```python
from build123d import *

# Parameters (mm, degrees)
CROQUIS1_W                = 139.5
CROQUIS1_H                = 83
SALIENTE_EXTRUIR1_DEPTH   = 27.5
CORTAR_EXTRUIR1_START     = -66.254131909
CORTAR_EXTRUIR1_OUTLINE_W = 22
CORTAR_EXTRUIR1_OUTLINE_H = 80
CORTAR_EXTRUIR1_DEPTH     = 132.508263818
CORTAR_EXTRUIR2_DEPTH     = 40
CROQUIS6_W                = 30
CROQUIS6_H                = 13.5
CROQUIS6_W_2              = 16.5
CORTAR_EXTRUIR3_DEPTH     = 3.495868091
CROQUIS7_R                = 2.5
CROQUIS7_W                = 21
CROQUIS7_H                = 30
CORTAR_EXTRUIR4_DEPTH     = 85.85207717


# Read off the part's stored shape, not the designer's step: Cortar-Extruir1
with BuildPart() as part:
    # Croquis1 → Saliente-Extruir1 (new body)
    with BuildSketch(Plane(origin=(0, 0, 0), x_dir=(1, 0, 0), z_dir=(0, 1, 0))):
        Rectangle(CROQUIS1_W, CROQUIS1_H)
    extrude(amount=SALIENTE_EXTRUIR1_DEPTH)

    # Cortar-Extruir1 outline → Cortar-Extruir1 (cut)
    with BuildSketch(Plane.YZ.offset(CORTAR_EXTRUIR1_START)):
        with Locations((13.75, -1.5)):
            Rectangle(CORTAR_EXTRUIR1_OUTLINE_W, CORTAR_EXTRUIR1_OUTLINE_H)
    extrude(amount=CORTAR_EXTRUIR1_DEPTH, mode=Mode.SUBTRACT)

    # Croquis3 → Cortar-Extruir2 (cut)
    with BuildSketch(Plane(origin=(0, 0, -41.5), x_dir=(-1, 0, 0), z_dir=(0, 0, -1))):
        Polygon((-66.254131909, 24.75), (67.373989774, 24.75), (69.75, 24.75), (69.75, 27.5), (67.373989774, 27.5), (-64.5, 27.5), (-69.75, 27.5), (-69.75, 23.25), (-69.75, 2.75), (-66.254131909, 2.75), align=None)
    extrude(amount=-CORTAR_EXTRUIR2_DEPTH, mode=Mode.SUBTRACT)

    # Croquis6 → Cortar-Extruir3 (cut)
    with BuildSketch(Plane(origin=(-66.254131909, 0, 0), x_dir=(0, 0, -1), z_dir=(1, 0, 0))):
        with Locations((-9.5, 9.5)):
            Rectangle(CROQUIS6_W, CROQUIS6_H)
        with Locations((18.75, 9.5)):
            Rectangle(CROQUIS6_W_2, CROQUIS6_H)
    extrude(amount=-CORTAR_EXTRUIR3_DEPTH, mode=Mode.SUBTRACT)

    # Croquis7 → Cortar-Extruir4 (cut, through all)
    with BuildSketch(Plane(origin=(0, 2.75, 0), x_dir=(1, 0, 0), z_dir=(0, 1, 0))):
        with Locations(Location((-58.754131909, 35.5, 0), (0, 0, 270))):
            Circle(CROQUIS7_R)
        with Locations(Location((60.25, 35.5, 0), (0, 0, 270))):
            Circle(CROQUIS7_R)
        with Locations((-59.25, -9.5)):
            Rectangle(CROQUIS7_W, CROQUIS7_H)
    extrude(amount=-CORTAR_EXTRUIR4_DEPTH, mode=Mode.SUBTRACT)


solid = part.part
```
Part model, mm, in its own coordinate system. A direction names the side the tool comes from. Round coordinates to 2 decimals unless told otherwise and drop trailing zeros. Write each loop counter-clockwise with the first axis right and the second up, starting at its lowest first coordinate (ties: lowest second). Pieces come first, ordered by that corner, then holes. Notation, with made-up numbers: M -27,54 L -2,54 A24 ccw -2,93 Z; hole C 53,44 d5. An arc over 180 degrees is marked long. Answer as CSV lines item,"result". Start each with the question number.
1) Band-saw the part on A-A (z = -35.5). List the corners of the cut face in (x, y).
2) Drop flat-ended pins along their axis: pin 1 (12.5 mm diameter, centred on x = -10, y = 10.5, fed in from -Z); pin 2 (4 mm diameter, centred on x = -68, z = -16.5, fed in from +Y); pin 3 (2 mm diameter, centred on x = -31.5, z = -15, fed in from +Y). Give the stop position or say it passes through.
3) Which spindle directions (+Z, -Z, +X, -X, +Y, -Y) get a long thin tool onto all of the face, cutting with end or side? Do faces 4 (the face through (-68, 9, -27)), 5 (the face through (-48.75, 1, 10)), 6 (the face through (-66.254, 18, -1)). Say none if no direction does.
4) Band-saw the part on C-C (y = 8.25). List the corners of the cut face in (x, z), then the cut area to 3 significant figures.
5) Drill centre lines: L1, parallel to X at y = 1.7, z = -35.5; L2, parallel to Y at x = -44.5, z = 8.5; L3, parallel to X at y = 21, z = 25.5. Where is each one in solid material? Low to high.
6) Band-saw the part on B-B (x = -54). List the corners of the cut face in (y, z), then the cut area to 3 significant figures.
7) Mould opens along Z. For faces 1 (the face through (-1, 14, 38.5)), 2 (the face through (-68, 24.75, -22)), 3 (the face through (-68, 16.25, 10)) say: +Z half, -Z half, draft (parallel to the pull), parting line (faces both ways), or undercut.
8) Band-saw the part on D-D (z = 2.5). List the corners of the cut face in (x, y).
Worked out:
1,outline,"M -69.75,0 L -61.25,0 L -61.25,2.75 L -66.25,2.75 L -66.25,24.75 L -69.75,24.75 Z; M -56.25,0 L 57.75,0 L 57.75,2.75 L -56.25,2.75 Z; M 62.75,0 L 69.75,0 L 69.75,2.75 L 62.75,2.75 Z"
2,pin 1,"z = 38.5"
2,pin 2,"y = 24.75"
2,pin 3,"y = 2.75"
3,face 4,"+X, -X"
3,face 5,"-X, -Y"
3,face 6,"-Z"
4,outline,"M -69.75,-41.5 L -66.25,-41.5 L -66.25,-27 L -69.75,-27 Z; M -69.75,-10.5 L -66.25,-10.5 L -66.25,-5.5 L -69.75,-5.5 Z; M -69.75,24.5 L -66.25,24.5 L -66.25,38.5 L 66.25,38.5 L 66.25,-1.5 L 69.75,-1.5 L 69.75,41.5 L -69.75,41.5 Z"
4,area,"675 mm²"
5,L1,"-69.75 to -61.25, -56.25 to 57.75, 62.75 to 69.75"
5,L2,"0 to 2.75, 24.75 to 27.5"
5,L3,"-69.75 to -66.25, 66.25 to 69.75"
6,outline,"M 0,-41.5 L 2.75,-41.5 L 2.75,-5.5 L 0,-5.5 Z; M 0,24.5 L 2.75,24.5 L 2.75,38.5 L 24.75,38.5 L 24.75,-1.5 L 27.5,-1.5 L 27.5,41.5 L 0,41.5 Z"
6,area,"330 mm²"
7,face 1,"-Z half"
7,face 2,"draft"
7,face 3,"undercut"
8,outline,"M -69.75,16.25 L -66.25,16.25 L -66.25,24.75 L 66.25,24.75 L 66.25,2.75 L -48.75,2.75 L -48.75,0 L 69.75,0 L 69.75,27.5 L -69.75,27.5 Z"
